Answer from the drawing. Dimensions are ordinates in mm from the lowest x, y and z of the part. Round coordinates to 2 decimals unless told otherwise and drop trailing zeros. Loops run counter-clockwise (first coordinate to the right, second up) from the corner with the lowest first, then second, coordinate; pieces in that order, holes last. Notation, with made-up numbers: M -23.75,-4.75 L 8.25,-4.75 A30 cw 8.25,20.25 Z; hole C -10,-4 d6. An arc over 180 degrees is marked long. One line per item, written item: value.
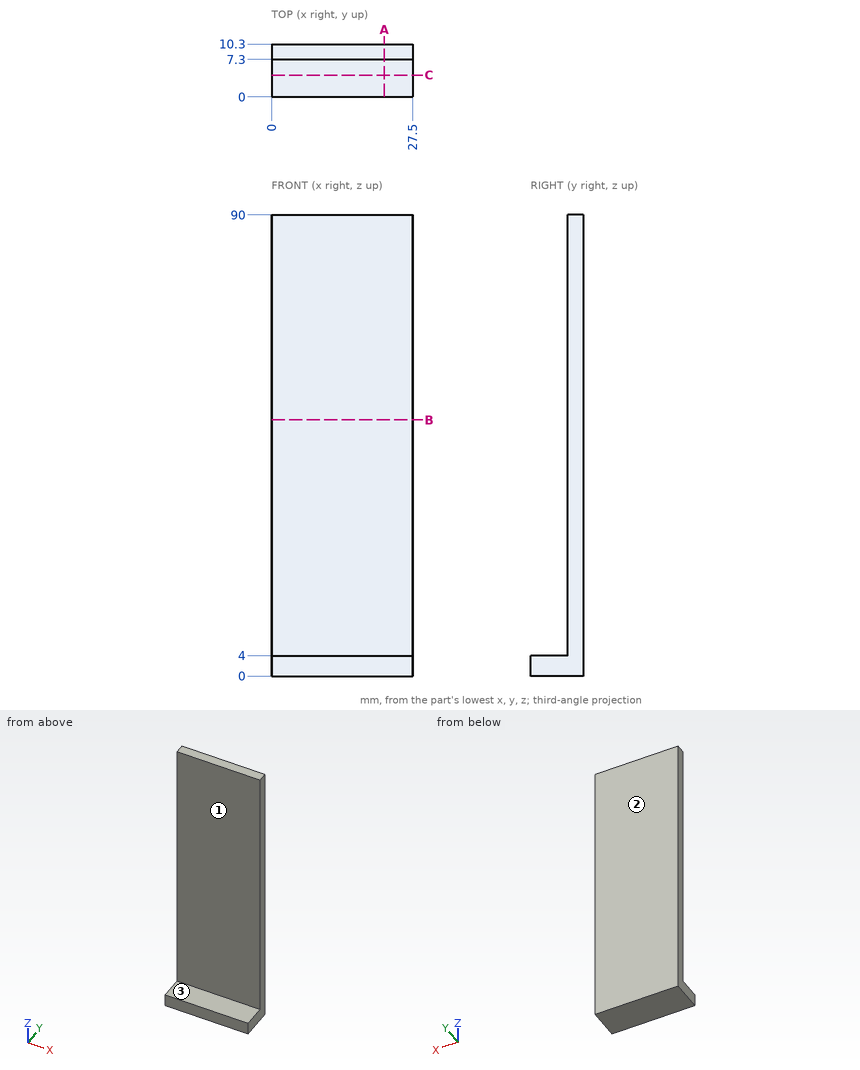
1) Find section A-A (x = 22). Give the vertices of the cut face in (y, z).
Check values:
outline: M 0,0 L 10.3,0 L 10.3,90 L 7.3,90 L 7.3,4 L 0,4 Z
2) Find section B-B (z = 50). Give the vertices of the cut face in (x, y).
Check values:
outline: M 0,7.3 L 27.5,7.3 L 27.5,10.3 L 0,10.3 Z
3) Find the intervals of material crossed by probe 1 along Z at (x, y) = (4, 6.25); probe 2 along Y at (x, z) = (8.25, 32.5), in increasing order. Write a range as from..to.
Check values:
probe 1: 0..4
probe 2: 7.3..10.3
4) The mould has two halves that part along Y. Classify the marked faces 1, 2 and 3: +Y half, -Y half, draft (parallel to the pull), parting line (faces both ways), or undercut.
Check values:
face 1: -Y half
face 2: +Y half
face 3: draft
5) Each of these flat-tipped pins is pushed along its axis until it touches: pin 1 (1 mm diameter, centred on x = 5, z = 49, fed in from -Y); pin 2 (1 mm diameter, centred on x = 4.5, y = 1.5, fed in from +Z). Where does it stop, or does it pass through?
Check values:
pin 1: y = 7.3
pin 2: z = 4
6) Find section C-C (y = 4.25). Give the vertices of the cut face in (x, z).
Check values:
outline: M 0,0 L 27.5,0 L 27.5,4 L 0,4 Z
